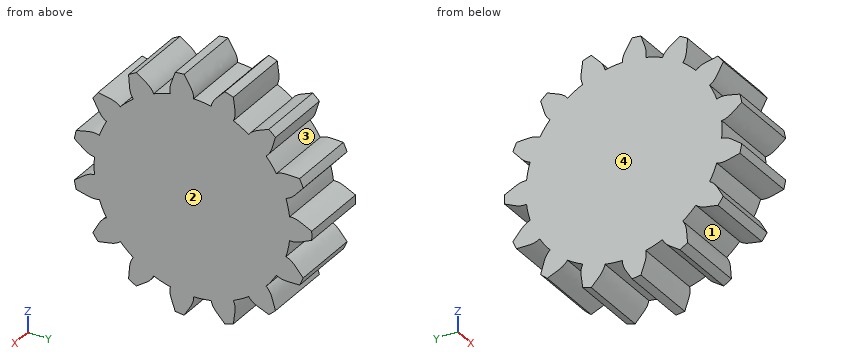
from build123d import *

# Parameters (mm, degrees)
BOSS_EXTRUDE1_DEPTH = 10
CIRPATTERN1_COUNT   = 15


with BuildPart() as part:
    # Sketch3 → Boss-Extrude1 (new body)
    with BuildSketch(Plane.YZ):
        with BuildLine():
            ThreePointArc((-1.141482098, 16.961633725), (-1.776983876, 16.906872221), (-2.409983971, 16.828308806))
            add(Edge.make_bspline(
                [(-2.409983971, 16.828308806), (-2.668426254, 15.877904884), (-3.400287418, 14.680650879), (-3.101338611, 13.595689764)],
                knots=[0.02683822, 0.02683822, 0.02683822, 0.02683822, 1.045667648, 1.045667648, 1.045667648, 1.045667648], degree=3))
            ThreePointArc((-3.101338611, 13.595689764), (1.457642136, -13.868538522), (0.206864074, 13.943395877))
            add(Edge.make_bspline(
                [(-1.141482098, 16.961633725), (-0.691087313, 16.085731582), (0.273704033, 15.066802941), (0.206864074, 13.943395877)],
                knots=[0.02683822, 0.02683822, 0.02683822, 0.02683822, 1.045667648, 1.045667648, 1.045667648, 1.045667648], degree=3))
        make_face()
    boss_extrude1 = extrude(amount=BOSS_EXTRUDE1_DEPTH)

    # CirPattern1: Boss-Extrude1 ×15 about axis
    cirpattern1_axis = Axis((10, 0, 0), (1, 0, 0))
    for i in range(1, CIRPATTERN1_COUNT):
        add(boss_extrude1.rotate(cirpattern1_axis, i * 360 / CIRPATTERN1_COUNT))


solid = part.part
Here's how the part is built. I have some questions about the finished solid (model axes, mm). Face numbers are marked on the shaded views. A direction names the side the tool comes from. Coordinates: 2 decimals unless noted, no trailing zeros. Order: outer loops, then holes, each group sorted by start corner. A loop starts at its lowest first (then second) coordinate and runs counter-clockwise, first axis right, second up. Notation, with made-up numbers: (6.5, 82) - (61.5, 82) arc R20 cw to (61.5, 98) - close; hole circle Ø2 at (82.25, 43). An arc over 180 degrees is marked (long way). Use CSV: the item, a comma, the result in double quotes. Start each with the question number.
1. I'm going to push flat-ended pins straight in: pin 1 (1.5 mm diameter, centred on x = 1.5, z = -12.5, fed in from +Y); pin 2 (1.5 mm diameter, centred on x = 4, z = -9.5, fed in from -Y); pin 3 (1 mm diameter, centred on y = 3, z = -6, fed in from -X). Where does each tip first touch, or does it pass through?
2. If we mould it in two halves opening along Z, with no side actions, what happens to the marked faces 1 and 2? For each: +Z half, -Z half, draft (parallel to the pull), parting line (faces both ways), or undercut.
3. Suppose I cut it at B-B on y = 2. List the corners of the cut face in (x, z) for me, then the cut area to 3 significant figures.
4. Please list where these lines run through material, in increasing order: line 1 (Z direction, x = 8.5, y = 15); line 2 (Z direction, x = 8.25, y = 13); line 3 (Y direction, x = 8.5, z = -12.5). Write a range as from..to.
5. Suppose I cut it at A-A on z = 0. List the corners of the cut face in (x, y) for me.
6. For the marked faces 3 and 4, which set-ups out of +Z, -Z, +X, -X, +Y, -Y let a thin tool reach every point of the face, with its end or its side?
Output:
1,pin 1,"stops at y = 11.84"
1,pin 2,"stops at y = -14.12"
1,pin 3,"stops at x = 0"
2,face 1,"undercut"
2,face 2,"draft"
3,outline,"(0, -13.8) - (10, -13.8) - (10, 13.8) - (0, 13.8) - close"
3,area,"276 mm2"
4,line 1,"z = -7.49..-5.41, -1.54..1.54, 5.41..7.49"
4,line 2,"z = -7.5..7.5"
4,line 3,"y = -8.89..6.18, 9.55..11.52"
5,outline,"(0, -13.94) - (10, -13.94) - (10, 17) - (0, 17) - close"
6,face 3,"+X, -X"
6,face 4,"+Z, -Z, -X, +Y, -Y"
